The listing builds one solid part. Answer for the finished solid, in the listing's coordinates (mm). Give positions to 0.01 mm unless a question says otherwise; leave off trailing zeros. Order: outer loops, then holes, each group sorted by start corner. A loop starts at its lowest first (then second) coordinate and runs counter-clockwise, first axis right, second up. Notation, with made-up numbers: (-18, -18) - (29, -18) arc R20 ccw to (29, -10) - close; hole circle Ø4 at (-13, -15.75). An arc over 180 degrees is marked (long way). Write each question's results on one line, items separated by ' | '. Start each with the question number.
1. Section B-B (z = 0.55) is taken. Give the vertices of the cut face in (x, y) (3 decimals).
2. Section C-C (x = 38.1) is taken. Give the vertices of the cut face in (y, z) (3 decimals), and give its area (3 significant figures).
3. Section A-A (y = 12.7) is taken. Give the vertices of the cut face in (x, z) (3 decimals).
4. Find the intervals of material crossed by L1, parallel to Y at x = 50.8, z = 1; L2, parallel to X at y = 11.75, z = 0.95; L3, parallel to Y at x = 37.5, z = 1.85, in increasing order.
5. Section D-D (x = 24) is taken. Give the vertices of the cut face in (y, z) (3 decimals).
Autodesk Inventor part; units mm, degrees
ref_plane "YZ Plane" through (0, 0, 0) normal (1, 0, 0) x (0, 1, 0)
ref_plane "XZ Plane" through (0, 0, 0) normal (0, 1, 0) x (-1, 0, 0)
ref_plane "XY Plane" through (0, 0, 0) normal (0, 0, 1) x (1, 0, 0)
sketch "Sketch1" plane through (0, 0, 0) normal (0, 0, 1) x (1, 0, 0)
  line L0 (0, 0) -> (76.2, 0)
  line L1 (76.2, 0) -> (76.2, 25.4)
  line L2 (76.2, 25.4) -> (0, 25.4)
  line L3 (0, 25.4) -> (0, 0)
  circle A0 centre (12.7, 12.7) radius 2.0828
  circle A1 centre (25.4, 12.7) radius 2.0828
  circle A2 centre (38.1, 12.7) radius 2.0828
  circle A3 centre (50.8, 12.7) radius 2.0828
  circle A4 centre (63.5, 12.7) radius 2.0828
  dimension "d0" = 76.2
  dimension "d1" = 25.4
  dimension "d2" = 4.1656
  dimension "d3" = 12.7
  dimension "d4" = 12.7
  dimension "d7" = 12.7
extrude "Extrusion1" add sketch "Sketch1" along normal blind 3.175
fillet "Fillet1" radius 3.175 4 edges at (0, 25.4, 1.5875) (0, 0, 1.5875) (76.2, 0, 1.5875) (76.2, 25.4, 1.5875)
properties part number "3 X 1 Spacer" material "Aluminum 6061"
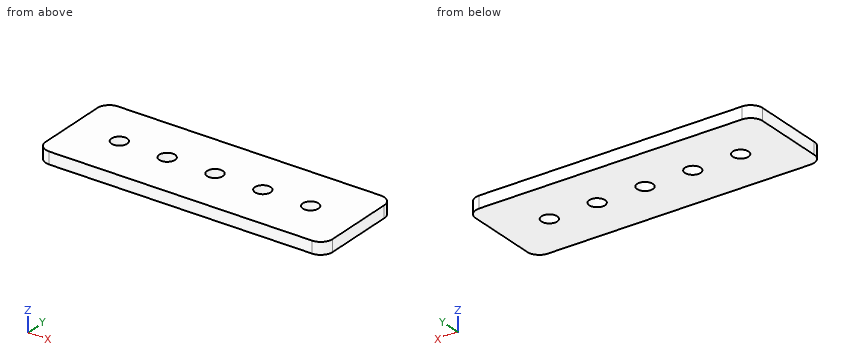
Reported:
1) outline: (0, 3.175) arc R3.175 ccw to (3.175, 0) - (73.025, 0) arc R3.175 ccw to (76.2, 3.175) - (76.2, 22.225) arc R3.175 ccw to (73.025, 25.4) - (3.175, 25.4) arc R3.175 ccw to (0, 22.225) - close; hole circle Ø4.166 at (12.7, 12.7); hole circle Ø4.166 at (25.4, 12.7); hole circle Ø4.166 at (38.1, 12.7); hole circle Ø4.166 at (50.8, 12.7); hole circle Ø4.166 at (63.5, 12.7)
2) outline: (0, 0) - (10.617, 0) - (10.617, 3.175) - (0, 3.175) - close; (14.783, 0) - (25.4, 0) - (25.4, 3.175) - (14.783, 3.175) - close | area: 67.4 mm²
3) outline: (0, 0) - (10.617, 0) - (10.617, 3.175) - (0, 3.175) - close; (14.783, 0) - (23.317, 0) - (23.317, 3.175) - (14.783, 3.175) - close; (27.483, 0) - (36.017, 0) - (36.017, 3.175) - (27.483, 3.175) - close; (40.183, 0) - (48.717, 0) - (48.717, 3.175) - (40.183, 3.175) - close; (52.883, 0) - (61.417, 0) - (61.417, 3.175) - (52.883, 3.175) - close; (65.583, 0) - (76.2, 0) - (76.2, 3.175) - (65.583, 3.175) - close
4) L1: 0 to 10.62, 14.78 to 25.4 | L2: 0 to 10.85, 14.55 to 23.55, 27.25 to 36.25, 39.95 to 48.95, 52.65 to 61.65, 65.35 to 76.2 | L3: 0 to 10.71, 14.69 to 25.4
5) outline: (0, 0) - (11.158, 0) - (11.158, 3.175) - (0, 3.175) - close; (14.242, 0) - (25.4, 0) - (25.4, 3.175) - (14.242, 3.175) - close
